```python
from build123d import *

# Parameters (mm, degrees)
BOSS_EXTRUDE2_DEPTH = 36


with BuildPart() as part:
    # Sketch1 → Boss-Extrude2 (new body)
    with BuildSketch(Plane.XY):
        with BuildLine():
            Line((-82, 0), (82, 0))
            Line((82, 0), (79, 11))
            Line((79, 11), (50, 11))
            Line((50, 11), (50, 54))
            Line((50, 54), (22, 54))
            Line((22, 54), (22, 41))
            Line((22, 41), (19, 41))
            Line((19, 41), (19, 38))
            ThreePointArc((19, 38), (0, 19), (-19, 38))
            Line((-19, 38), (-19, 41))
            Line((-19, 41), (-22, 41))
            Line((-22, 41), (-22, 54))
            Line((-22, 54), (-50, 54))
            Line((-50, 54), (-50, 11))
            Line((-50, 11), (-79, 11))
            Line((-79, 11), (-82, 0))
        make_face()
    extrude(amount=BOSS_EXTRUDE2_DEPTH)


solid = part.part
```
Can you work these out from the model? Positions are in its coordinate system, mm. A direction names the side the tool comes from. Coordinates: 2 decimals unless noted, no trailing zeros. Loops run counter-clockwise (first coordinate to the right, second up) from the corner with the lowest first, then second, coordinate; pieces in that order, holes last.
Item 1: I'm going to push flat-ended pins straight in: pin 1 (3.5 mm diameter, centred on x = 20, z = 13.5, fed in from +Y); pin 2 (2 mm diameter, centred on y = 33.5, z = 11, fed in from +X); pin 3 (0.9 mm diameter, centred on y = 39.5, z = 27, fed in from -X). Where does each tip first touch, or does it pass through?
Answers below:
pin 1: stops at y = 41
pin 2: stops at x = 50
pin 3: stops at x = -50
Item 2: Suppose I cut it at D-D (y = 15). Please give me the cut outline in (x, z).
Answers below:
outline: (-50, 0) - (50, 0) - (50, 36) - (-50, 36) - close
Item 3: Which directions (+Z, -Z, +X, -X, +Y, -Y) give clear straight access to the entire face, cutting with the end or side of a thin tool? Please do faces 5 (the face through (65, 11, 18)), 6 (the face through (-22, 47, 18)), 7 (the face through (-64, 11, 18)), 8 (the face through (-1, 15, 0)).
Answers below:
face 5: +Z, -Z, +X, +Y
face 6: +Z, -Z, +Y
face 7: +Z, -Z, -X, +Y
face 8: -Z, +X, -X, +Y, -Y
Item 4: If we mould it in two halves opening along X, with no side actions, what happens to faces 1 (the face through (-20, 41, 18)), 2 (the face through (21, 41, 18)), 3 (the face through (50, 32, 18)), 4 (the face through (-1, 0, 18))? For each: released by +X, released by -X, zero draft, split by the parting line, or undercut.
Answers below:
face 1: undercut
face 2: undercut
face 3: released by +X
face 4: zero draft
Item 5: Suppose I cut it at A-A (y = 31.5). Please give me the cut outline in (x, z), then the cut area to 3 significant figures.
Answers below:
outline: (-50, 0) - (-17.85, 0) - (-17.85, 36) - (-50, 36) - close; (17.85, 0) - (50, 0) - (50, 36) - (17.85, 36) - close
area: 2,310 mm2
Item 6: Suppose I cut it at C-C (x = 0). Please give me the cut outline in (y, z).
Answers below:
outline: (0, 0) - (19, 0) - (19, 36) - (0, 36) - close
Item 7: Please list where these lines run through material, in increasing order: L1, parallel to X at y = 51.5, z = 13.5; L2, parallel to Y at x = -56, z = 6; L3, parallel to X at y = 39.5, z = 9.5.
Answers below:
L1: x = -50 to -22, 22 to 50
L2: y = 0 to 11
L3: x = -50 to -19, 19 to 50
Item 8: Suppose I cut it at B-B (z = 9). Please give me the cut outline in (x, y), then the cut area to 3 significant figures.
Answers below:
outline: (-82, 0) - (82, 0) - (79, 11) - (50, 11) - (50, 54) - (22, 54) - (22, 41) - (19, 41) - (19, 38) arc R19 cw to (-19, 38) - (-19, 41) - (-22, 41) - (-22, 54) - (-50, 54) - (-50, 11) - (-79, 11) - close
area: 4,820 mm2
